The model under review builds one solid part; all positions refer to its coordinate system, in mm. Face numbers are marked on the shaded views. A direction names the side the tool comes from. Coordinates: 2 decimals unless noted, no trailing zeros. Order: outer loops, then holes, each group sorted by start corner. A loop starts at its lowest first (then second) coordinate and runs counter-clockwise, first axis right, second up. Notation, with made-up numbers: M 22,-33 L 80,-33 A25 cw 80,-7 Z; hole C 71,-16 d7. An arc over 180 degrees is marked long. One line per item, written item: value.
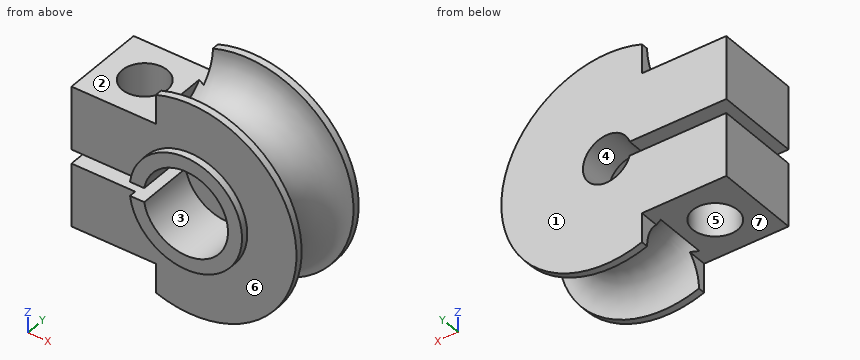
```python
from build123d import *

# Parameters (mm, degrees)
CLAMP_EXTRUSION_DEPTH      = 5
CLAMP_EXTRUSION_DEPTH_BACK = 5
SKETCH2_W                  = 5.5
SKETCH2_H                  = 6
SKETCH3_W                  = 6
SKETCH3_H                  = 2.071067812
SKETCH3_W_2                = 8.5
SKETCH3_H_2                = 1
CLAMP_CUTOUT_DEPTH         = 14.067134468
CLAMP_HOLE_D               = 3.2


with BuildPart() as part:
    # Sketch1 → body (revolve)
    with BuildSketch(Plane.XY, mode=Mode.PRIVATE) as body_sk:
        with BuildLine():
            Line((3, 0), (4, 0))
            Line((4, 0), (4, 0.5))
            Line((4, 0.5), (7.5, 0.5))
            Line((7.5, 0.5), (7.5, 1))
            ThreePointArc((7.5, 1), (5, 3.5), (7.5, 6))
            Line((7.5, 6), (7.5, 6.5))
            Line((7.5, 6.5), (1.7, 6.5))
            Line((1.7, 6.5), (1.7, 4))
            Line((1.7, 4), (3, 4))
            Line((3, 4), (3, 0))
        make_face()
    revolve(body_sk.sketch.rotate(Axis((0, 0, 0), (0, 1, 0)), 90), axis=Axis((0, 0, 0), (0, 1, 0)))

    # Sketch2 → clamp_extrusion (add, two sides: drawn at the far end of the back side and taken through both)
    with BuildSketch(Plane.XY.offset(-CLAMP_EXTRUSION_DEPTH_BACK)):
        with Locations((-5.75, 3.5)):
            Rectangle(SKETCH2_W, SKETCH2_H)
    extrude(amount=CLAMP_EXTRUSION_DEPTH + CLAMP_EXTRUSION_DEPTH_BACK)

    # Sketch3 → clamp_cutout (cut, through all)
    with BuildSketch(Plane(origin=(0, 6.5, 0), x_dir=(1, 0, 0), z_dir=(0, 1, 0))):
        with Locations((-5.5, 6.035533906)):
            Rectangle(SKETCH3_W, SKETCH3_H)
        with Locations((-5.5, -6.035533906)):
            Rectangle(SKETCH3_W, SKETCH3_H)
        with Locations((-4.25, 0)):
            Rectangle(SKETCH3_W_2, SKETCH3_H_2)
    extrude(amount=-CLAMP_CUTOUT_DEPTH, mode=Mode.SUBTRACT)

    # clamp_hole (through all)
    with Locations(Plane.XY.offset(5)):
        with Locations((-5.5, 3.5)):
            Hole(CLAMP_HOLE_D / 2)


solid = part.part
```
(1) For L1, parallel to X at y = 3.75, z = 0.75; L2, parallel to X at y = 2.25, z = -1.5; L3, parallel to Z at x = -5, y = 5.75, list the stretches that pass through material, from the lowest coordinate up.
Geometry results:
L1: x = -8.5 to -7.08, -3.92 to -2.9, 2.9 to 4.96
L2: x = -8.5 to -6.5, -4.5 to -2.6, 2.6 to 5.12
L3: z = -5 to -0.5, 0.5 to 5
(2) Tool access review of the marked faces 5, 6 and 7: name each direction out of +Z, -Z, +X, -X, +Y, -Y from which nothing blocks a thin tool from reaching the whole face with its end or side.
Geometry results:
face 5: +Z, -Z
face 6: -Y
face 7: -Z, -X, +Y, -Y
(3) Mouldability with a two-part tool opening along Z and no side actions: class the marked faces 1, 2, 3 and 4 as +Z half, -Z half, draft (parallel to the pull), parting line (faces both ways), or undercut.
Geometry results:
face 1: draft
face 2: +Z half
face 3: undercut
face 4: undercut
(4) We need section C-C, the plane x = -5.5. State the section outline as (y, z) points, plus the area to 3 significant figures.
Geometry results:
outline: M 0.5,-5 L 1.9,-5 L 1.9,-0.5 L 0.5,-0.5 Z; M 0.5,0.5 L 1.9,0.5 L 1.9,5 L 0.5,5 Z; M 5.1,-5 L 6.5,-5 L 6.5,-0.5 L 5.1,-0.5 Z; M 5.1,0.5 L 6.5,0.5 L 6.5,5 L 5.1,5 Z
area: 25.2 mm2
(5) We need section A-A, the plane x = 0. State the section outline as (y, z) points.
Geometry results:
outline: M 0,-4 L 0.5,-4 L 0.5,-7.5 L 1,-7.5 A2.5 cw 6,-7.5 L 6.5,-7.5 L 6.5,-1.7 L 4,-1.7 L 4,-3 L 0,-3 Z; M 0,3 L 4,3 L 4,1.7 L 6.5,1.7 L 6.5,7.5 L 6,7.5 A2.5 cw 1,7.5 L 0.5,7.5 L 0.5,4 L 0,4 Z
(6) We need section B-B, the plane y = 3.5. State the section outline as (x, z) points, plus the area to 3 significant figures.
Geometry results:
outline: M -8.5,-5 L -7.1,-5 L -7.1,-0.5 L -8.5,-0.5 Z; M -8.5,0.5 L -7.1,0.5 L -7.1,5 L -8.5,5 Z; M -3.9,-5 L -3,-5 L -3,-4 A5 ccw long -3,4 L -3,5 L -3.9,5 L -3.9,0.5 L -2.96,0.5 A3 cw long -2.96,-0.5 L -3.9,-0.5 Z
area: 59.8 mm2
(7) Insertion check: pin 1 Ø7.5 at (x, z) = (0.5, -1.5) entering from -Y; pin 2 Ø1.5 at (y, z) = (1, -6.5) entering from -X; pin 3 Ø2 at (y, z) = (4, 3.5) entering from +X; pin 4 Ø1.1 at (y, z) = (2.5, -4.5) entering from +X. Each pin has a flat end and moves straight along its axis. Give the tip position at first contact, or say it passes through.
Geometry results:
pin 1: stops at y = 0
pin 2: stops at x = -2.5
pin 3: stops at x = 4.52
pin 4: stops at x = 3.54
(8) We need section D-D, the plane z = 0. State the section outline as (x, y) points.
Geometry results:
outline: M 1.7,4 L 3,4 L 3,0 L 4,0 L 4,0.5 L 7.5,0.5 L 7.5,1 A2.5 cw 7.5,6 L 7.5,6.5 L 1.7,6.5 Z
